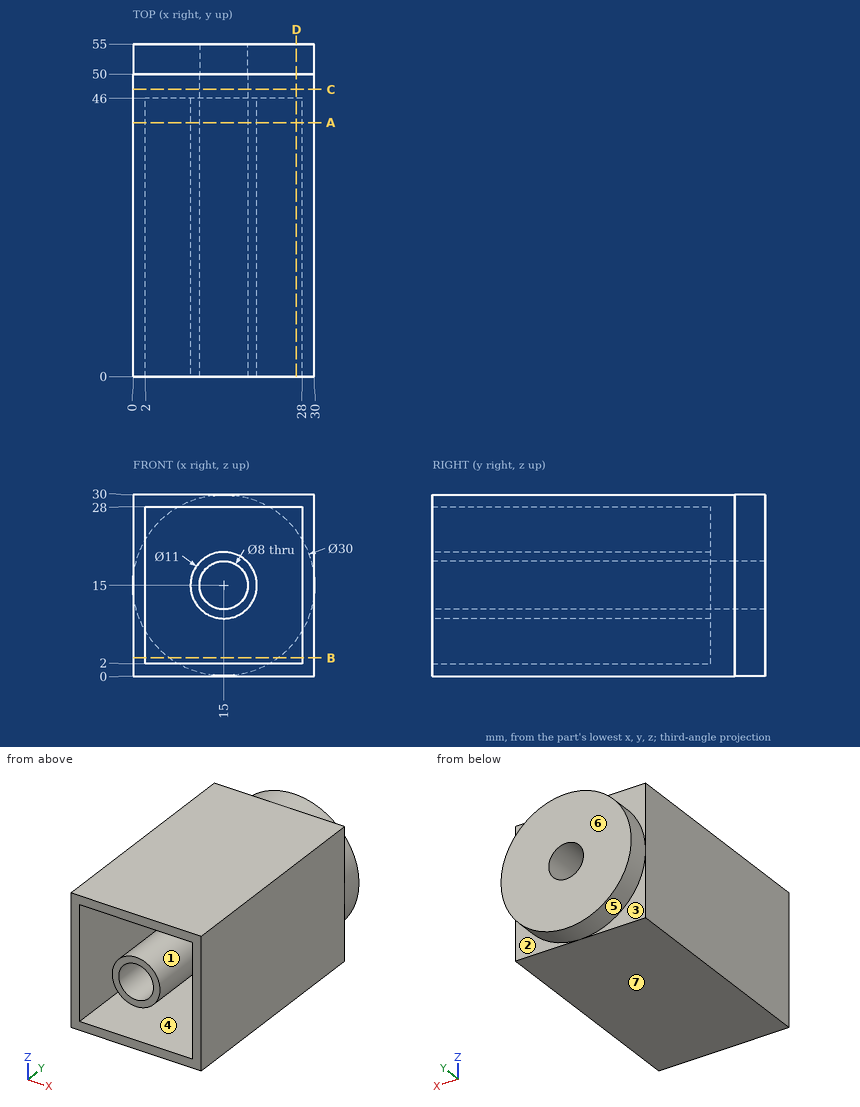
For this review, use the dimensioned drawing (mm, ordinates from the lowest corner) and the shaded views. A direction names the side the tool comes from. Give positions to 0.01 mm unless a question says otherwise; leave off trailing zeros. Order: outer loops, then holes, each group sorted by start corner. A loop starts at its lowest first (then second) coordinate and runs counter-clockwise, first axis right, second up. Notation, with made-up numbers: (46.25, -30.75) - (72.25, -30.75) arc R10 cw to (72.25, -23.75) - close; hole circle Ø3 at (47, -24). An arc over 180 degrees is marked (long way). Write item = value, one per line. Start each with the question number.
Q1. To check wall thickness, follow L1, parallel to Z at x = 15, y = 39; L2, parallel to X at y = 28, z = 23.5. State the ranges of each line that lie inside material, in increasing order. Write a range as from..to.
Q2. We need section B-B on z = 3. State the section outline as (x, y) points.
Q3. We need section D-D on x = 27. State the section outline as (y, z) points.
Q4. Clearance check with a flat-ended pin moving along its axis: pin 1 Ø1.5 at (x, z) = (3, 14) entering from -Y. State where the tip first meets the part, or that it passes through.
Q5. Mouldability with a two-part tool opening along Z and no side actions: class the marked faces 4, 5, 6 and 7 as released by +Z, released by -Z, zero draft, split by the parting line, or undercut.
Q6. We need section C-C on y = 47.5. State the section outline as (x, z) points, plus the area to 3 significant figures.
Q7. Tool access review of the marked faces 1, 2 and 3: name each direction out of +Z, -Z, +X, -X, +Y, -Y from which nothing blocks a thin tool from reaching the whole face with its end or side.
Q8. We need section A-A on y = 42. State the section outline as (x, z) points.
Working result:
q1.L1 = 0..2, 9.5..11, 19..20.5, 28..30
q1.L2 = 0..2, 28..30
q2.outline = (0, 0) - (2, 0) - (2, 46) - (28, 46) - (28, 0) - (30, 0) - (30, 50) - (24, 50) - (24, 55) - (6, 55) - (6, 50) - (0, 50) - close
q3.outline = (0, 0) - (50, 0) - (50, 6) - (55, 6) - (55, 24) - (50, 24) - (50, 30) - (0, 30) - (0, 28) - (46, 28) - (46, 2) - (0, 2) - close
q4.pin_1 = 46
q5.face_4 = undercut
q5.face_5 = split by the parting line
q5.face_6 = zero draft
q5.face_7 = released by -Z
q6.outline = (0, 0) - (30, 0) - (30, 30) - (0, 30) - close; hole circle Ø8 at (15, 15)
q6.area = 850 mm²
q7.face_1 = -Y
q7.face_2 = -Z, +X, +Y
q7.face_3 = -Z, -X, +Y
q8.outline = (0, 0) - (30, 0) - (30, 30) - (0, 30) - close; circle Ø11 at (15, 15); hole (2, 2) - (28, 2) - (28, 28) - (2, 28) - close; hole circle Ø8 at (15, 15)
